```python
from build123d import *

# Parameters (mm, degrees)
SKETCH1_W                      = 793.75
SKETCH1_H                      = 63.5
BASE_FLANGE1_DEPTH             = 2.05232
EDGE_FLANGE1_STRIP_W           = 13.28928
EDGE_FLANGE1_STRIP_H           = 2.05232
EDGE_FLANGE1_STRIP_CUT_DEPTH   = 793.75
EDGE_FLANGE1_STRIP_2_W         = 13.28928
EDGE_FLANGE1_STRIP_2_H         = 2.05232
EDGE_FLANGE1_STRIP_CUT_2_DEPTH = 793.75
EDGE_FLANGE1_DEPTH             = 793.75
EDGE_FLANGE1_BEND_DEPTH        = 793.75
F_10_0_1935_DIAMETER_HOLE1_D   = 4.9149
BREAK_CORNER1_START            = -65.55232
BREAK_CORNER1_DEPTH            = 67.60464
F_1_4_CLEARANCE_HOLE1_D        = 6.7564


# Read off the part's stored shape, not the designer's step: Break-Corner1
# Sheet-metal steps are written as plain solids
with BuildPart() as part:
    # Sketch1 → Base-Flange1 (new body)
    with BuildSketch(Plane(origin=(0, 0, 0), x_dir=(1, 0, 0), z_dir=(0, 1, 0))):
        with Locations((396.875, 31.75)):
            Rectangle(SKETCH1_W, SKETCH1_H)
    extrude(amount=-BASE_FLANGE1_DEPTH)

    # Edge-Flange1 strip (across the edge) → Edge-Flange1 strip cut (cut)
    with BuildSketch(Plane(origin=(0, 0, 0), x_dir=(0, 0, -1), z_dir=(1, 0, 0))):
        with Locations((-4.10464, -1.02616)):
            Rectangle(EDGE_FLANGE1_STRIP_W, EDGE_FLANGE1_STRIP_H)
    extrude(amount=EDGE_FLANGE1_STRIP_CUT_DEPTH, mode=Mode.SUBTRACT)

    # Edge-Flange1 strip 2 (across the edge) → Edge-Flange1 strip cut 2 (cut)
    with BuildSketch(Plane(origin=(793.75, 0, -63.5), x_dir=(0, 0, 1), z_dir=(-1, 0, 0))):
        with Locations((-4.10464, -1.02616)):
            Rectangle(EDGE_FLANGE1_STRIP_2_W, EDGE_FLANGE1_STRIP_2_H)
    extrude(amount=EDGE_FLANGE1_STRIP_CUT_2_DEPTH, mode=Mode.SUBTRACT)

    # Edge-Flange1 section (across the edge) → Edge-Flange1 (add)
    with BuildSketch(Plane(origin=(0, 0, 0), x_dir=(0, 0, -1), z_dir=(1, 0, 0))):
        with BuildLine():
            Line((-2.05232, 2.54), (-2.05232, 55.09768))
            Line((-2.05232, 55.09768), (0, 55.09768))
            Line((0, 55.09768), (0, 2.54))
            ThreePointArc((0, 2.54), (0.743948776, 0.743948776), (2.54, 0))
            Line((2.54, 0), (2.54, -2.05232))
            ThreePointArc((2.54, -2.05232), (-0.707260613, -0.707260613), (-2.05232, 2.54))
        make_face()
    extrude(amount=EDGE_FLANGE1_DEPTH)

    # Edge-Flange1 section 2 (across the edge) → Edge-Flange1 bend (add)
    with BuildSketch(Plane(origin=(793.75, 0, -63.5), x_dir=(0, 0, 1), z_dir=(-1, 0, 0))):
        with BuildLine():
            Line((-2.05232, 2.54), (-2.05232, 55.09768))
            Line((-2.05232, 55.09768), (0, 55.09768))
            Line((0, 55.09768), (0, 2.54))
            ThreePointArc((0, 2.54), (0.743948776, 0.743948776), (2.54, 0))
            Line((2.54, 0), (2.54, -2.05232))
            ThreePointArc((2.54, -2.05232), (-0.707260613, -0.707260613), (-2.05232, 2.54))
        make_face()
    extrude(amount=EDGE_FLANGE1_BEND_DEPTH)

    # #10 (0.1935) Diameter Hole1 (through all)
    with Locations(Plane.XY.offset(2.05232)):
        with Locations((12.7, 42.39768), (12.7, 16.99768), (44.45, 42.39768), (44.45, 16.99768), (749.3, 16.99768), (781.05, 16.99768), (781.05, 42.39768), (749.3, 42.39768)):
            Hole(F_10_0_1935_DIAMETER_HOLE1_D / 2)

    # Break-Corner1 outline → Break-Corner1 (cut)
    with BuildSketch(Plane.XY.offset(BREAK_CORNER1_START)):
        with BuildLine():
            ThreePointArc((0, 48.74768), (1.859871939, 53.237808061), (6.35, 55.09768))
            Line((6.35, 55.09768), (0, 55.09768))
            Line((0, 55.09768), (0, 48.74768))
        make_face()
        with BuildLine():
            ThreePointArc((787.4, 55.09768), (791.890128061, 53.237808061), (793.75, 48.74768))
            Line((793.75, 48.74768), (793.75, 55.09768))
            Line((793.75, 55.09768), (787.4, 55.09768))
        make_face()
    extrude(amount=BREAK_CORNER1_DEPTH, mode=Mode.SUBTRACT)

    # 1/4 Clearance Hole1 (through all)
    with Locations(Plane(origin=(0, 0, 0), x_dir=(1, 0, 0), z_dir=(0, 1, 0))):
        with Locations((219.075, 31.75), (574.675, 31.75), (25.4, 31.75), (768.35, 31.75)):
            Hole(F_1_4_CLEARANCE_HOLE1_D / 2)


solid = part.part
```
The model under review builds one solid part; all positions refer to its coordinate system, in mm. A direction names the side the tool comes from. Round coordinates to 2 decimals unless told otherwise and drop trailing zeros. Write each loop counter-clockwise with the first axis right and the second up, starting at its lowest first coordinate (ties: lowest second). Pieces come first, ordered by that corner, then holes. Notation, with made-up numbers: (-38.5, 35) - (2.5, 35) arc R14 ccw to (2.5, 41) - close; hole circle Ø7 at (10.25, -19). An arc over 180 degrees is marked (long way). Answer as CSV lines item,"result". Start each with the question number.
(1) Draft analysis for pull direction Z (two halves, no side actions). For faces 1 (the flat face through (391, 29, 0)), 2 (the flat face through (402, 29, -63.5)), 3 (the flat face through (793.75, -1, -32)), 4 (the flat face through (402, 28, -65.552)), state which applies: pulls with the +Z half, pulls with the -Z half, needs draft (parallel to the pull), parting line crosses it, or undercut.
(2) To check wall thickness, follow line 1 (X direction, y = -1.3, z = -31.75); line 2 (Z direction, x = 600.5, y = 31.5); line 3 (Y direction, x = 12.7, z = 0.85). State the ranges of each line that lie inside material, in increasing order.
(3) We need section A-A on x = 399.5. State the section outline as (y, z) points, plus the area to 3 significant figures.
(4) For faces 5 (the flat face through (391, 0, -32)), 6 (the flat face through (391, -2.052, -32)), list the 3-axis set-ups (+Z, -Z, +X, -X, +Y, -Y) from which the entire face can be reached by the end or side of a thin tool; tool diameter is ignored.
(5) For pin 1 Ø3 at (x, y) = (12.7, 42.4) entering from +Z; pin 2 Ø8 at (x, z) = (574.675, -31.75) entering from +Y, all flat-tipped, find the tip position at first contact; note any pin that passes through.
Worked answers:
1,face 1,"undercut"
1,face 2,"undercut"
1,face 3,"needs draft"
1,face 4,"pulls with the -Z half"
2,line 1,"0 to 22.02, 28.78 to 215.7, 222.45 to 571.3, 578.05 to 764.97, 771.73 to 793.75"
2,line 2,"-65.55 to -63.5, 0 to 2.05"
2,line 3,"-0.56 to 14.54, 19.46 to 39.94, 44.86 to 55.1"
3,outline,"(-2.05, -60.96) arc R4.59 ccw to (2.54, -65.55) - (55.1, -65.55) - (55.1, -63.5) - (2.54, -63.5) arc R2.54 cw to (0, -60.96) - (0, -2.54) arc R2.54 cw to (2.54, 0) - (55.1, 0) - (55.1, 2.05) - (2.54, 2.05) arc R4.59 ccw to (-2.05, -2.54) - close"
3,area,"359 mm²"
4,face 5,"+X, -X, +Y"
4,face 6,"+Z, -Z, +X, -X, -Y"
5,pin 1,"through"
5,pin 2,"y = 0"
